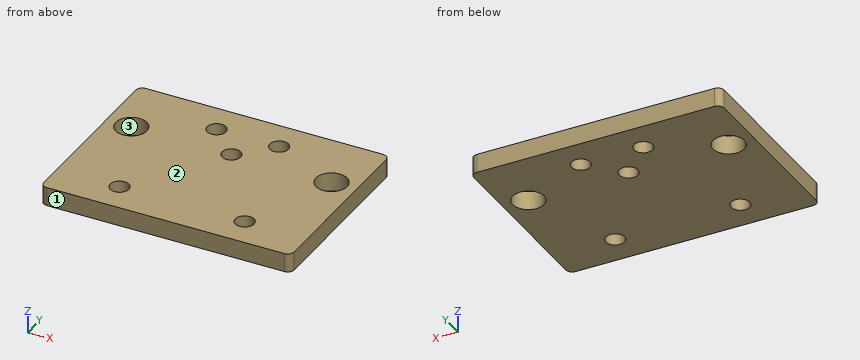
from build123d import *

# Parameters (mm, degrees)
SKETCH_1_W          = 40
SKETCH_1_H          = 20
SKETCH_1_R          = 2.5
EXTRUDE_1_DEPTH     = 3
SKETCH_2_R          = 1.5
CUT_EXTRUDE_1_DEPTH = 3
SKETCH_4_W          = 40
SKETCH_4_H          = 10
EXTRUDE_2_DEPTH     = 3
SKETCH_5_R          = 1.5
CUT_EXTRUDE_2_DEPTH = 10
SKETCH_6_R          = 1.5
CUT_EXTRUDE_3_DEPTH = 10
FILLET_1_R          = 1


with BuildPart() as part:
    # 草图1 → 凸台-拉伸1 (new body)
    with BuildSketch(Plane.XY):
        Rectangle(SKETCH_1_W, SKETCH_1_H)
        with Locations((-16, 0)):
            Circle(SKETCH_1_R, mode=Mode.SUBTRACT)
        with Locations((16, 0)):
            Circle(SKETCH_1_R, mode=Mode.SUBTRACT)
    extrude(amount=EXTRUDE_1_DEPTH)

    # 草图2 → 切除-拉伸1 (cut)
    with BuildSketch(Plane.XY.offset(3)):
        Circle(SKETCH_2_R)
    extrude(amount=-CUT_EXTRUDE_1_DEPTH, mode=Mode.SUBTRACT)

    # 草图4 → 凸台-拉伸2 (add)
    with BuildSketch(Plane.XY.offset(3)):
        with Locations((0, -15)):
            Rectangle(SKETCH_4_W, SKETCH_4_H)
    extrude(amount=-EXTRUDE_2_DEPTH)

    # 草图5 → 切除-拉伸2 (cut)
    with BuildSketch(Plane.XY.offset(3)):
        with Locations((-10, -15)):
            Circle(SKETCH_5_R)
        with Locations((10, -15)):
            Circle(SKETCH_5_R)
    extrude(amount=-CUT_EXTRUDE_2_DEPTH, mode=Mode.SUBTRACT)

    # 草图6 → 切除-拉伸3 (cut)
    with BuildSketch(Plane.XY.offset(3)):
        with Locations((-5, 5)):
            Circle(SKETCH_6_R)
        with Locations((5, 5)):
            Circle(SKETCH_6_R)
    extrude(amount=-CUT_EXTRUDE_3_DEPTH, mode=Mode.SUBTRACT)

    # 圆角1
    fillet_1_edges = [part.edges().sort_by_distance(p)[0] for p in [
        (-20, -20, 1.5),
        (20, -20, 1.5),
        (-20, 10, 1.5),
        (20, 10, 1.5),
    ]]
    fillet(fillet_1_edges, radius=FILLET_1_R)


solid = part.part
Could you check a few things on this model? Use its own coordinates, in mm. Face numbers are marked on the shaded views. Give positions to 0.01 mm unless a question says otherwise; leave off trailing zeros. Order: outer loops, then holes, each group sorted by start corner. A loop starts at its lowest first (then second) coordinate and runs counter-clockwise, first axis right, second up.
1. Suppose I cut it at C-C (z = 1.2). List the corners of the cut face in (x, y) for me.
2. Will this pin go through, and if not, where does the flat tip stop? P1, Ø4, axis at x = -16, y = 0, coming from the +Z side.
3. I need wall thicknesses on L1, parallel to Y at x = 5, z = 1.2; L2, parallel to Y at x = 14, z = 1.9; L3, parallel to X at y = 4.75, z = 2.8. Which ranges of each line are inside material? Lowest first, please.
4. Suppose I cut it at D-D (y = 0). List the corners of the cut face in (x, z) for me, plus the area to 3 significant figures.
5. Suppose I cut it at A-A (x = 0). List the corners of the cut face in (y, z) for me.
6. We'd pull the mould along Y, two halves only. Please class the marked faces 1, 2 and 3: pulls with the +Y half, pulls with the -Y half, needs draft (parallel to the pull), parting line crosses it, or undercut.
7. Suppose I cut it at B-B (y = 5). List the corners of the cut face in (x, z) for me.
Solved:
1. outline: (-20, -19) arc R1 ccw to (-19, -20) - (19, -20) arc R1 ccw to (20, -19) - (20, 9) arc R1 ccw to (19, 10) - (-19, 10) arc R1 ccw to (-20, 9) - close; hole circle Ø5 at (-16, 0); hole circle Ø3 at (-10, -15); hole circle Ø3 at (-5, 5); hole circle Ø3 at (0, 0); hole circle Ø3 at (5, 5); hole circle Ø3 at (10, -15); hole circle Ø5 at (16, 0)
2. P1: passes through
3. L1: y = -20 to 3.5, 6.5 to 10
3. L2: y = -20 to -1.5, 1.5 to 10
3. L3: x = -20 to -6.48, -3.52 to 3.52, 6.48 to 20
4. outline: (-20, 0) - (-18.5, 0) - (-18.5, 3) - (-20, 3) - close; (-13.5, 0) - (-1.5, 0) - (-1.5, 3) - (-13.5, 3) - close; (1.5, 0) - (13.5, 0) - (13.5, 3) - (1.5, 3) - close; (18.5, 0) - (20, 0) - (20, 3) - (18.5, 3) - close
4. area: 81.0 mm2
5. outline: (-20, 0) - (-1.5, 0) - (-1.5, 3) - (-20, 3) - close; (1.5, 0) - (10, 0) - (10, 3) - (1.5, 3) - close
6. face 1: pulls with the -Y half
6. face 2: needs draft
6. face 3: undercut
7. outline: (-20, 0) - (-6.5, 0) - (-6.5, 3) - (-20, 3) - close; (-3.5, 0) - (3.5, 0) - (3.5, 3) - (-3.5, 3) - close; (6.5, 0) - (20, 0) - (20, 3) - (6.5, 3) - close
